Build history of the part. All positions in model axes, mm. A direction names the side the tool comes from. Give positions to 0.01 mm unless a question says otherwise; leave off trailing zeros. Loops run counter-clockwise (first coordinate to the right, second up) from the corner with the lowest first, then second, coordinate; pieces in that order, holes last. Notation, with made-up numbers: (-15, -11) -> (27, -11) arc R27 ccw to (27, 27) -> close; hole circle Ø7 at (9.5, 68.25). An arc over 180 degrees is marked (long way). Answer in a Markdown table with one row per item. Add a question column.
from build123d import *

# Parameters (mm, degrees)
BOSS_EXTRUDE1_DEPTH     = 12.7
RIB3_START              = -3.175
RIB3_DEPTH              = 3.175
CUT_EXTRUDE3_DEPTH      = 102.649597269
CUT_EXTRUDE3_DEPTH_BACK = 102.649597269
CUT_EXTRUDE4_DEPTH      = 102.649597269
SKETCH6_W               = 25.4
SKETCH6_H               = 12.7
BOSS_EXTRUDE2_DEPTH     = 19.05
CUT_EXTRUDE5_DEPTH      = 19.05
SKETCH9_W               = 22.86
SKETCH9_H               = 25.4
CUT_EXTRUDE6_DEPTH      = 2.54
FILLET4_R               = 3.175
FILLET5_R               = 6.35


# Read off the part's stored shape, not the designer's step: Rib3
with BuildPart() as part:
    # Sketch1 → Boss-Extrude1 (new, symmetric)
    with BuildSketch(Plane.XY):
        Polygon((-47.625, 0), (47.625, 0), (47.625, 6.35), (19.05, 6.35), (19.05, 88.9), (12.7, 88.9), (12.7, 6.35), (-12.7, 6.35), (-12.7, 88.9), (-19.05, 88.9), (-19.05, 6.35), (-47.625, 6.35), align=None)
    extrude(amount=BOSS_EXTRUDE1_DEPTH, both=True)

    # Rib3 outline → Rib3 (add)
    with BuildSketch(Plane(origin=(0, 0, -12.7), x_dir=(-1, 0, 0), z_dir=(0, 0, -1)).offset(RIB3_START)):
        Polygon((-19.05, 88.9), (-22.225, 88.9), (-47.625, 6.35), (-19.05, 6.35), align=None)
    rib3 = extrude(amount=RIB3_DEPTH)

    # Mirror1: Rib3 across plane
    add(rib3.mirror(Plane(origin=(0, 0, 0), x_dir=(0, 0, 1), z_dir=(1, 0, 0))))

    # Sketch4 → Cut-Extrude3 (cut, two sides: drawn at the far end of the back side and taken through both)
    with BuildSketch(Plane(origin=(0, 0, 0), x_dir=(0, 0, -1), z_dir=(1, 0, 0)).offset(-CUT_EXTRUDE3_DEPTH_BACK)):
        with BuildLine():
            Line((2.38125, 63.5), (2.38125, 25.4))
            ThreePointArc((2.38125, 25.4), (-1.5875, 21.43125), (-5.55625, 25.4))
            Line((-5.55625, 25.4), (-5.55625, 63.5))
            ThreePointArc((-5.55625, 63.5), (-1.5875, 67.46875), (2.38125, 63.5))
        make_face()
    extrude(amount=CUT_EXTRUDE3_DEPTH + CUT_EXTRUDE3_DEPTH_BACK, mode=Mode.SUBTRACT)

    # Sketch5 → Cut-Extrude4 (cut, through all)
    with BuildSketch(Plane.XZ):
        with BuildLine():
            Line((-42.8625, 3.175), (-33.3375, 3.175))
            ThreePointArc((-33.3375, 3.175), (-30.1625, 0), (-33.3375, -3.175))
            Line((-33.3375, -3.175), (-42.8625, -3.175))
            ThreePointArc((-42.8625, -3.175), (-46.0375, 0), (-42.8625, 3.175))
        make_face()
        with BuildLine():
            Line((42.8625, -3.175), (33.3375, -3.175))
            ThreePointArc((33.3375, -3.175), (30.1625, 0), (33.3375, 3.175))
            Line((33.3375, 3.175), (42.8625, 3.175))
            ThreePointArc((42.8625, 3.175), (46.0375, 0), (42.8625, -3.175))
        make_face()
    extrude(amount=-CUT_EXTRUDE4_DEPTH, mode=Mode.SUBTRACT)

    # Sketch6 → Boss-Extrude2 (add)
    with BuildSketch(Plane.ZY.offset(19.05)):
        with Locations((0, 82.55)):
            Rectangle(SKETCH6_W, SKETCH6_H)
    extrude(amount=BOSS_EXTRUDE2_DEPTH)

    # Sketch7 → Cut-Extrude5 (cut)
    with BuildSketch(Plane(origin=(0, 88.9, 0), x_dir=(1, 0, 0), z_dir=(0, 1, 0))):
        with BuildLine():
            Line((-30.48, -4.0005), (-43.18, -4.0005))
            ThreePointArc((-43.18, -4.0005), (-45.593, -1.5875), (-43.18, 0.8255))
            Line((-43.18, 0.8255), (-30.48, 0.8255))
            ThreePointArc((-30.48, 0.8255), (-28.067, -1.5875), (-30.48, -4.0005))
        make_face()
    extrude(amount=-CUT_EXTRUDE5_DEPTH, mode=Mode.SUBTRACT)

    # Sketch9 → Cut-Extrude6 (cut)
    with BuildSketch(Plane(origin=(0, 88.9, 0), x_dir=(1, 0, 0), z_dir=(0, 1, 0))):
        with Locations((-24.13, 0)):
            Rectangle(SKETCH9_W, SKETCH9_H)
    extrude(amount=-CUT_EXTRUDE6_DEPTH, mode=Mode.SUBTRACT)

    # Fillet4
    fillet4_edges = [part.edges().sort_by_distance(p)[0] for p in [
        (-38.1, 76.2, -6.76275),
        (-38.1, 76.2, 8.35025),
        (12.7, 88.9, 0),
        (-12.7, 86.36, 0),
        (22.225, 88.9, -11.1125),
    ]]
    fillet(fillet4_edges, radius=FILLET4_R)

    # Fillet5
    fillet5_edges = [part.edges().sort_by_distance(p)[0] for p in [
        (-26.132692308, 76.2, -11.1125),
        (-19.05, 76.2, 1.5875),
        (-19.05, 6.35, 1.5875),
        (-12.7, 6.35, 0),
        (12.7, 6.35, 0),
        (19.05, 6.35, 1.5875),
    ]]
    fillet(fillet5_edges, radius=FILLET5_R)


solid = part.part
(1) Flat gauge pins, fed straight in: pin 1 Ø2 at (y, z) = (19, 2) entering from +X; pin 2 Ø12.5 at (y, z) = (61, 3) entering from -X; pin 3 Ø1 at (x, y) = (-30, 56.5) entering from +Z (3 decimals); pin 4 Ø1.5 at (x, y) = (37, 45.5) entering from +Z. Where does each tip first touch, or does it go through?
(2) Saw through at A-A, the plane y = 58. List the corners of the cut face in (x, z) (3 decimals), then the cut area to 3 significant figures.
(3) Saw through at C-C, the plane y = 71. List the corners of the cut face in (x, z) (3 decimals), then the cut area to 3 significant figures.
(4) Saw through at B-B, the plane x = 40.5. List the corners of the cut face in (y, z) (3 decimals), then the cut area to 3 significant figures.
(5) Wall check: line 1 along X through (y, z) = (43, -7); line 2 along Y through (x, z) = (37.5, 5.25). Give the ranges that are in metal, low to high. Write a range as from..to.
(6) Two-plate mould, pull along Y, no slides. Class faces 1 (the cylindrical face through (-37.19, 77.15, 8.41)), 2 (the flat face through (0, 6.35, 0)), 3 (the flat face through (-38, 3, 3.175)): released by +Y, released by -Y, zero draft, split by the parting line, or undercut.
(7) Saw through at D-D, the plane z = 7.25. List the corners of the cut face in (x, y) (3 decimals).
(8) 3-axis set-ups, long thin cutter, end or side, ignore diameter. For faces 4 (the cylindrical face through (-15.919, 21.432, 1.5)), 5 (the flat face through (-34, 81, -0.826)), 6 (the flat face through (-34, 81, 4)), 7 (the cylindrical face through (46.037, 3.131, 0.07)), 8 (the flat face through (-35.56, 88, -7)): which of +Z, -Z, +X, -X, +Y, -Y reach the whole face in a straight line?
Worked answers:
| question | item | result |
|---|---|---|
| 1 | pin 1 | x = 19.05 |
| 1 | pin 2 | x = -19.05 |
| 1 | pin 3 | z = -9.525 |
| 1 | pin 4 | through |
| 2 | outline | (-31.733, -12.7) -> (-12.7, -12.7) -> (-12.7, -2.381) -> (-19.05, -2.381) -> (-19.05, -9.525) -> (-31.733, -9.525) -> close; (-19.05, 5.556) -> (-12.7, 5.556) -> (-12.7, 12.7) -> (-19.05, 12.7) -> close; (12.7, -12.7) -> (31.733, -12.7) -> (31.733, -9.525) -> (19.05, -9.525) -> (19.05, -2.381) -> (12.7, -2.381) -> close; (12.7, 5.556) -> (19.05, 5.556) -> (19.05, 12.7) -> (12.7, 12.7) -> close |
| 2 | area | 302 mm^2 |
| 3 | outline | (-28.485, -12.7) -> (-12.7, -12.7) -> (-12.7, 12.7) -> (-19.155, 12.7) -> (-19.155, -9.525) -> (-28.485, -9.525) -> close; (12.7, -12.7) -> (27.733, -12.7) -> (27.733, -9.525) -> (19.05, -9.525) -> (19.05, 12.7) -> (12.7, 12.7) -> close |
| 3 | area | 382 mm^2 |
| 4 | outline | (0, -12.7) -> (29.506, -12.7) -> (29.506, -9.525) -> (6.35, -9.525) -> (6.35, -3.175) -> (0, -3.175) -> close; (0, 3.175) -> (6.35, 3.175) -> (6.35, 12.7) -> (0, 12.7) -> close |
| 4 | area | 194 mm^2 |
| 5 | line 1 | -19.05..-12.7, 12.7..19.05 |
| 5 | line 2 | 0..6.35 |
| 6 | face 1 | undercut |
| 6 | face 2 | released by +Y |
| 6 | face 3 | zero draft |
| 7 | outline | (-47.625, 0) -> (47.625, 0) -> (47.625, 6.35) -> (25.4, 6.35) arc R6.35 cw to (19.05, 12.7) -> (19.05, 88.9) -> (15.875, 88.9) arc R3.175 ccw to (12.7, 85.725) -> (12.7, 12.7) arc R6.35 cw to (6.35, 6.35) -> (-6.35, 6.35) arc R6.35 cw to (-12.7, 12.7) -> (-12.7, 83.185) arc R3.175 ccw to (-15.875, 86.36) -> (-35.56, 86.36) -> (-35.56, 88.9) -> (-38.1, 88.9) -> (-38.1, 79.375) arc R3.175 ccw to (-34.925, 76.2) -> (-25.4, 76.2) arc R6.35 cw to (-19.05, 69.85) -> (-19.05, 12.7) arc R6.35 cw to (-25.4, 6.35) -> (-47.625, 6.35) -> close |
| 8 | face 4 | +X, -X |
| 8 | face 5 | -X, +Y, -Y |
| 8 | face 6 | -X, +Y |
| 8 | face 7 | +Y, -Y |
| 8 | face 8 | +Z, -Z, +Y |
